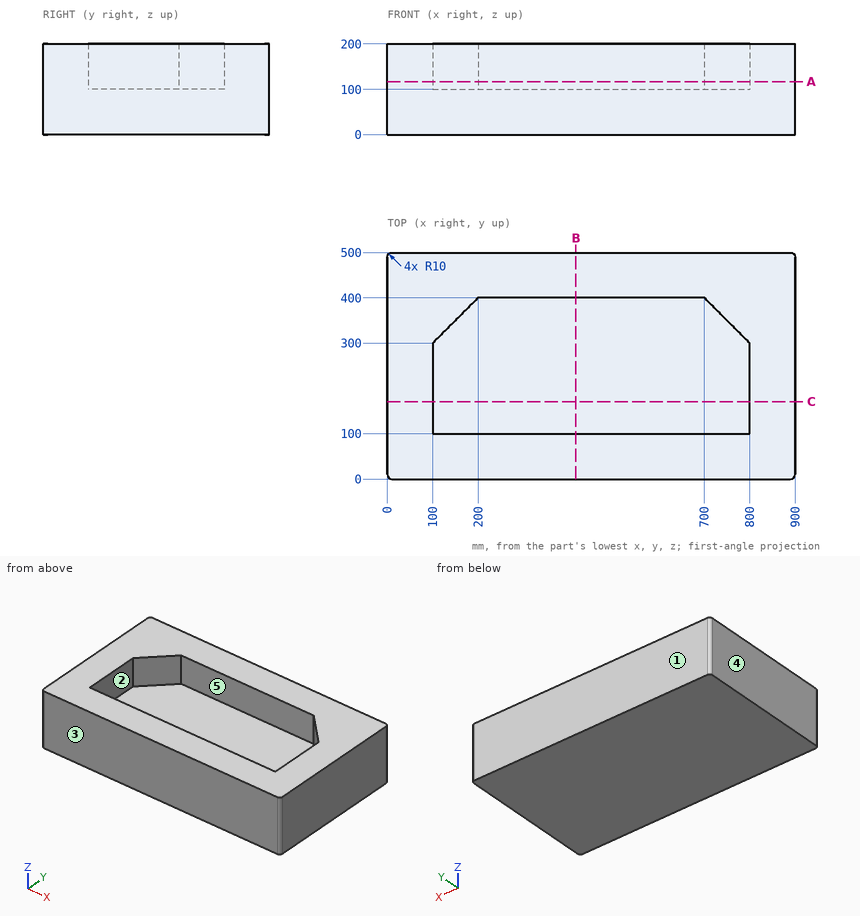
Design review of the part shown in the three views and the two pictorial views. Dimensions are in mm from the part's minimum x, y and z. A direction names the side the tool comes from. Give positions to 0.01 mm unless a question says otherwise; leave off trailing zeros. Write each loop counter-clockwise with the first axis right and the second up, starting at its lowest first coordinate (ties: lowest second). Pieces come first, ordered by that corner, then holes.
(1) Wall thickness on line 1 along Y through (x, z) = (588, 109); line 2 along X through (y, z) = (194.5, 179); line 3 along Z through (x, y) = (214, 151): over which ranges is each line inside the solid? List them lowest first.
Checked values:
line 1: y = 0 to 100, 400 to 500
line 2: x = 0 to 100, 800 to 900
line 3: z = 0 to 100
(2) Add section A-A (z = 117). Give the boundary of the cut face in (x, y).
Checked values:
outline: (0, 10) arc R10 ccw to (10, 0) - (890, 0) arc R10 ccw to (900, 10) - (900, 490) arc R10 ccw to (890, 500) - (10, 500) arc R10 ccw to (0, 490) - close; hole (100, 100) - (800, 100) - (800, 300) - (700, 400) - (200, 400) - (100, 300) - close
(3) Add section B-B (x = 416). Give the boundary of the cut face in (y, z).
Checked values:
outline: (0, 0) - (500, 0) - (500, 200) - (400, 200) - (400, 100) - (100, 100) - (100, 200) - (0, 200) - close
(4) Mouldability with a two-part tool opening along X and no side actions: class the marked faces 3, 4 and 5 as +X half, -X half, draft (parallel to the pull), parting line (faces both ways), or undercut.
Checked values:
face 3: draft
face 4: -X half
face 5: undercut
(5) Tool access review of the marked faces 1 and 2: name each direction out of +Z, -Z, +X, -X, +Y, -Y from which nothing blocks a thin tool from reaching the whole face with its end or side.
Checked values:
face 1: +Z, -Z, +X, -X, +Y
face 2: +Z
(6) Add section C-C (y = 171). Give the boundary of the cut face in (x, z), and give its area (3 significant figures).
Checked values:
outline: (0, 0) - (900, 0) - (900, 200) - (800, 200) - (800, 100) - (100, 100) - (100, 200) - (0, 200) - close
area: 110,000 mm2
